Work out the finished part from the listing and answer in its coordinate system (mm). Coordinates: 2 decimals unless noted, no trailing zeros. Order: outer loops, then holes, each group sorted by start corner. A loop starts at its lowest first (then second) coordinate and runs counter-clockwise, first axis right, second up. Notation, with made-up numbers: (44, 63.5) -> (88, 63.5) arc R22 ccw to (88, 81.5) -> close; hole circle Ø1 at (26, -10.75). An arc over 180 degrees is marked (long way). Use one line per item in the form item = value.
from build123d import *

# Parameters (mm, degrees)
F0_W     = 152.4
F0_H     = 76.2
F0_R     = 12.7
F1_DEPTH = 38.1


with BuildPart() as f1:
    # F0 (on Front) → F1 (new body)
    with BuildSketch(Plane.XZ):
        Rectangle(F0_W, F0_H)
        with Locations((-38.1, 0)):
            Circle(F0_R, mode=Mode.SUBTRACT)
        with BuildLine():
            ThreePointArc((50.8, 0), (38.1, -12.7), (25.4, 0))
            ThreePointArc((25.4, 0), (38.1, 12.7), (50.8, 0))
        make_face(mode=Mode.SUBTRACT)
    extrude(amount=F1_DEPTH)


solid = f1.part
(1) Section A-A on x = -38.1 is taken. Write down the section's boundary in (y, z).
Data:
outline = (-38.1, -38.1) -> (0, -38.1) -> (0, -12.7) -> (-38.1, -12.7) -> close; (-38.1, 12.7) -> (0, 12.7) -> (0, 38.1) -> (-38.1, 38.1) -> close
(2) This flat-tipped pin is pushed along its axis until it touches: P1, Ø15, axis at x = 38.1, z = 0, coming from the +Y side. Where does it stop, or does it pass through?
Data:
P1 = through
(3) Straight lines are drawn through the part: line 1 along Z through (x, y) = (-38.1, -9.5); line 2 along X through (y, z) = (-1.5, 8); line 3 along X through (y, z) = (-31, -6.5). For each, find the intervals that lie inside material, in ascending order.
Data:
line_1 = -38.1 to -12.7, 12.7 to 38.1
line_2 = -76.2 to -47.96, -28.24 to 28.24, 47.96 to 76.2
line_3 = -76.2 to -49.01, -27.19 to 27.19, 49.01 to 76.2
(4) Section C-C on y = -3 is taken. Write down the section's boundary in (x, z).
Data:
outline = (-76.2, -38.1) -> (76.2, -38.1) -> (76.2, 38.1) -> (-76.2, 38.1) -> close; hole circle Ø25.4 at (-38.1, 0); hole circle Ø25.4 at (38.1, 0)
(5) Section B-B on z = 0 is taken. Write down the section's boundary in (x, y).
Data:
outline = (-76.2, -38.1) -> (-50.8, -38.1) -> (-50.8, 0) -> (-76.2, 0) -> close; (-25.4, -38.1) -> (25.4, -38.1) -> (25.4, 0) -> (-25.4, 0) -> close; (50.8, -38.1) -> (76.2, -38.1) -> (76.2, 0) -> (50.8, 0) -> close
(6) The mould has two halves that part along X. Classify faces 1 (the cylindrical face through (50.788, -18.783, 0.558)), 2 (the flat face through (-1, -38.1, 1)), 3 (the flat face through (76.2, -19, -1)), 4 (the cylindrical face through (-48.2, -18.8, -7.7)): released by +X, released by -X, zero draft, split by the parting line, or undercut.
Data:
face_1 = undercut
face_2 = zero draft
face_3 = released by +X
face_4 = undercut
